For this review, take the finished solid that the model builds, in its own axes (mm). A direction names the side the tool comes from. Give positions to 0.01 mm unless a question says otherwise; leave off trailing zeros. Return JSON: item names as keys, results as strings.
from build123d import *

# Parameters (mm, degrees)
BLANKSKE_W          = 180
BLANKSKE_H          = 17.25
BLANK_DEPTH         = 7
TOOTHCUTSIM_DEPTH   = 181.960113008
TEETHCUTS_COUNT     = 26
TEETHCUTS_PITCH     = 7.068583463
SKETCH1_W           = 7
SKETCH1_H           = 12.1875
BOSS_EXTRUDE1_DEPTH = 12.5


with BuildPart() as part:
    # BlankSke → Blank (new body)
    with BuildSketch(Plane.XY):
        with Locations((90, 8.625)):
            Rectangle(BLANKSKE_W, BLANKSKE_H)
    extrude(amount=-BLANK_DEPTH)

    # TooCutSkeSim → ToothCutSim (cut, through all)
    with BuildSketch(Plane.XY):
        Polygon((0.974479582, 12.1875), (-0.974479582, 12.1875), (-2.826323737, 17.2754), (2.826323737, 17.2754), align=None)
    toothcutsim = extrude(amount=-TOOTHCUTSIM_DEPTH, mode=Mode.SUBTRACT)

    # TeethCuts: ToothCutSim ×26
    with Locations(*[(i * TEETHCUTS_PITCH, 0, 0) for i in range(1, TEETHCUTS_COUNT)]):
        add(toothcutsim, mode=Mode.SUBTRACT)

    # Sketch1 → Boss-Extrude1 (add)
    with BuildSketch(Plane.ZY):
        with Locations((-3.5, 6.09375)):
            Rectangle(SKETCH1_W, SKETCH1_H)
    extrude(amount=BOSS_EXTRUDE1_DEPTH)


solid = part.part
1. To check wall thickness, follow probe 1 along Y at (x, z) = (43, -1.75). State the ranges of the line that lie inside material, in increasing order.
Results found:
{"probe 1": "y = 0 to 12.19"}
2. For faces 1 (the flat face through (40.53, 14.68, -3.45)), 2 (the flat face through (-12.5, 6, -4)), 3 (the flat face through (-6, 12.188, -4)), list the 3-axis set-ups (+Z, -Z, +X, -X, +Y, -Y) from which the entire face can be reached by the end or side of a thin tool; tool diameter is ignored.
Results found:
{"face 1": "+Z, -Z, +Y", "face 2": "+Z, -Z, -X, +Y, -Y", "face 3": "+Z, -Z, -X, +Y"}
3. For pin 1 (1.6 mm diameter, centred on x = 42.5, z = -2, fed in from +Y), flat-tipped, find the tip position at first contact; note if it passes through.
Results found:
{"pin 1": "stops at y = 12.19"}
